from build123d import *

# Parameters (mm, degrees)
BASEHEAD_DEPTH   = 7.76
INDENT_OUTLINE_R = 7.875
INDENT_DEPTH     = 0.97
SKETCH4_W        = 0.6
SKETCH4_H        = 11.392304845


# Read off the part's stored shape, not the designer's step: Indent
with BuildPart() as part:
    # Sketch1 → BaseHead (new body)
    with BuildSketch(Plane(origin=(0, 0, 0), x_dir=(0, 0, -1), z_dir=(1, 0, 0))):
        Polygon((9, 5.196152423), (9, -5.196152423), (0, -10.392304845), (-9, -5.196152423), (-9, 5.196152423), (0, 10.392304845), align=None)
    extrude(amount=BASEHEAD_DEPTH)

    # BodySke → BaseBody (revolve)
    with BuildSketch(Plane.XY, mode=Mode.PRIVATE) as basebody_sk:
        Polygon((0, 0), (87.76, 0), (87.76, 5.036), (86.796, 6), (0, 6), align=None)
    revolve(basebody_sk.sketch.rotate(Axis((0, 0, 0), (1, 0, 0)), 90), axis=Axis((0, 0, 0), (1, 0, 0)))

    # Indent outline → Indent (cut)
    with BuildSketch(Plane.YZ):
        with Locations((0.192376607, 0.033212245)):
            Circle(INDENT_OUTLINE_R)
    extrude(amount=INDENT_DEPTH, mode=Mode.SUBTRACT)

    # Sketch3 → HeadChamfer (revolve, cut)
    with BuildSketch(Plane.XY):
        Polygon((0, 9), (3.690598923, 15.392304845), (3.690598923, 20.392304845), (-10, 20.392304845), (-10, 9), align=None)
    revolve(axis=Axis((0, 0, 0), (1, 0, 0)), mode=Mode.SUBTRACT)

    # Sketch4 → BearingFace (revolve, cut)
    with BuildSketch(Plane.XY, mode=Mode.PRIVATE) as bearingface_sk:
        with Locations((7.46, 14.696152423)):
            Rectangle(SKETCH4_W, SKETCH4_H)
    revolve(bearingface_sk.sketch.rotate(Axis((0, 0, 0), (1, 0, 0)), 270), axis=Axis((0, 0, 0), (1, 0, 0)), mode=Mode.SUBTRACT)


solid = part.part
Build history of the part. All positions in model axes, mm. A direction names the side the tool comes from. Round coordinates to 2 decimals unless told otherwise and drop trailing zeros. Write each loop counter-clockwise with the first axis right and the second up, starting at its lowest first coordinate (ties: lowest second). Pieces come first, ordered by that corner, then holes. Notation, with made-up numbers: (76, 9.25) -> (86, 9.25) arc R12 cw to (86, 13.25) -> close; hole circle Ø10 at (14, 18). An arc over 180 degrees is marked (long way). Write item = value, one per line.
(1) Two-plate mould, pull along Y, no slides. Class faces 5 (the face through (0.97, 0, 0)), 6 (the face through (3.53, 7.76, 4.56)), 7 (the face through (4, 0, 9)), 8 (the face through (0.2, -4.69, -8.08)): pulls with the +Y half, pulls with the -Y half, needs draft (parallel to the pull), parting line crosses it, or undercut.
Answer:
face_5 = undercut
face_6 = pulls with the +Y half
face_7 = needs draft
face_8 = pulls with the -Y half
(2) Tool access for faces 1 (the face through (7.16, -5, -8)), 2 (the face through (7.16, 4.5, 8.1)), 3 (the face through (7.16, 4.5, -8.1)), 4 (the face through (7.46, -5.48, 7.14)): list every direction of +Z, -Z, +X, -X, +Y, -Y with a clear straight run to the whole face (end or side of a thin tool).
Answer:
face_1 = -Z, +X, -Y
face_2 = +Z, +X, +Y
face_3 = -Z, +X, +Y
face_4 = +X
(3) Flat gauge pins, fed straight in: pin 1 (10 mm diameter, centred on x = 14, z = -2, fed in from +Y); pin 2 (2 mm diameter, centred on y = -5, z = -6.5, fed in from +X); pin 3 (10 mm diameter, centred on x = 39, y = 6.5, fed in from +Z); pin 4 (1.5 mm diameter, centred on y = -6.5, z = 5, fed in from -X). Where does each tip first touch, or does it go through?
Answer:
pin_1 = 6
pin_2 = 7.76
pin_3 = 5.81
pin_4 = 0
(4) Band-saw the part on A-A (x = 49). Give the cut face in (y, z).
Answer:
outline = circle Ø12 at (0, 0)
(5) Probe L1, parallel to X at y = 0.75, z = 2.5; L2, parallel to X at y = 2.5, z = 8; L3, parallel to Y at x = 70, z = -3. List the from-to ranges inside material, lowest first.
Answer:
L1 = 0.97 to 87.76
L2 = 0 to 7.76
L3 = -5.2 to 5.2
